Read the model definition and answer for the solid it produces. Units are mm, in the model's axes. A direction names the side the tool comes from. Give positions to 0.01 mm unless a question says otherwise; leave off trailing zeros. Write each loop counter-clockwise with the first axis right and the second up, starting at its lowest first coordinate (ties: lowest second). Pieces come first, ordered by that corner, then holes. Notation, with made-up numbers: (34, 47) -> (50, 47) arc R27 ccw to (50, 68) -> close; hole circle Ø10 at (78.25, 26.25). An arc over 180 degrees is marked (long way). Use a Markdown table: item, result.
from build123d import *

# Parameters (mm, degrees)
SKETCH2_R           = 2.5
BOSS_EXTRUDE1_DEPTH = 3
CUT_EXTRUDE1_START  = -15
CUT_EXTRUDE1_DEPTH  = 15


with BuildPart() as part:
    # Sketch1 → Revolve1 (revolve)
    with BuildSketch(Plane.XY, mode=Mode.PRIVATE) as revolve1_sk:
        Polygon((0, 48.5), (37.1, 48.5), (37.1, 4), (82.1, 4), (82.1, 2.5), (94.1, 2.5), (94.1, 0), (-101.4, 0), (-101.4, 2.4), (-89.4, 2.4), (-89.4, 4), (-38.4, 4), (-38.4, 48.5), align=None)
    revolve(revolve1_sk.sketch.rotate(Axis((0, 0, 0), (-1, 0, 0)), 90), axis=Axis((0, 0, 0), (-1, 0, 0)))

    # Sketch2 → Boss-Extrude1 (add)
    with BuildSketch(Plane(origin=(0, 0, 0), x_dir=(0, 0, -1), z_dir=(1, 0, 0))):
        with BuildLine():
            Line((-7.930604102, 69.771502825), (-16.421800454, 47.75536064))
            ThreePointArc((-16.421800454, 47.75536064), (-43.734282891, 25.25), (-49.568255708, -9.655983951))
            Line((-49.568255708, -9.655983951), (-64.389195958, -28.017646793))
            ThreePointArc((-64.389195958, -28.017646793), (-65.136215932, -37.606411802), (-56.458591856, -41.753856033))
            Line((-56.458591856, -41.753856033), (-33.146455254, -38.099376689))
            ThreePointArc((-33.146455254, -38.099376689), (0, -50.5), (33.146455254, -38.099376689))
            Line((33.146455254, -38.099376689), (56.458591856, -41.753856033))
            ThreePointArc((56.458591856, -41.753856033), (65.136215932, -37.606411802), (64.389195958, -28.017646793))
            Line((64.389195958, -28.017646793), (49.568255708, -9.655983951))
            ThreePointArc((49.568255708, -9.655983951), (43.734282891, 25.25), (16.421800454, 47.75536064))
            Line((16.421800454, 47.75536064), (7.930604102, 69.771502825))
            ThreePointArc((7.930604102, 69.771502825), (0, 75.212823605), (-7.930604102, 69.771502825))
        make_face()
        with Locations((0, 66.712823605)):
            Circle(SKETCH2_R, mode=Mode.SUBTRACT)
        with Locations((57.775, -33.356411802)):
            Circle(SKETCH2_R, mode=Mode.SUBTRACT)
        with Locations((-57.775, -33.356411802)):
            Circle(SKETCH2_R, mode=Mode.SUBTRACT)
    extrude(amount=BOSS_EXTRUDE1_DEPTH)

    # Sketch4 → Cut-Extrude1 (cut)
    with BuildSketch(Plane.ZY.offset(89.4).offset(CUT_EXTRUDE1_START)):
        with BuildLine():
            Line((-2.645751311, 3), (2.645751311, 3))
            ThreePointArc((2.645751311, 3), (0, 4), (-2.645751311, 3))
        make_face()
    extrude(amount=CUT_EXTRUDE1_DEPTH, mode=Mode.SUBTRACT)


solid = part.part
Item 1: Straight lines are drawn through the part: line 1 along X through (y, z) = (19, 17.5); line 2 along X through (y, z) = (-31, 45); line 3 along Z through (x, y) = (33, 38). For each, find the intervals that lie inside material, in ascending order. Write a range as [from, to].
Return value:
| item | result |
|---|---|
| line 1 | [-38.4, 37.1] |
| line 2 | [0, 3] |
| line 3 | [-30.14, 30.14] |
Item 2: A cutting plane is placed at C-C (z = 40). Give the vertices of the cut face in (x, y).
Return value:
| item | result |
|---|---|
| outline | (-38.4, -27.43) -> (0, -27.43) -> (0, -39.17) -> (3, -39.17) -> (3, -27.43) -> (37.1, -27.43) -> (37.1, 27.43) -> (3, 27.43) -> (3, 30.83) -> (0, 30.83) -> (0, 27.43) -> (-38.4, 27.43) -> close |
Item 3: Each of these flat-tipped pins is pushed along its axis until it touches: P1, Ø4.5, axis at y = 66.71, z = 0, coming from the +X side; P2, Ø8, axis at y = -33.36, z = 57.78, coming from the -X side; P3, Ø12, axis at x = 40.5, z = 45.5, coming from the +Y side; P4, Ø4, axis at x = -85, z = -0.5, coming from the +Y side. Where does it stop, or does it pass through?
Return value:
| item | result |
|---|---|
| P1 | through |
| P2 | x = 0 |
| P3 | y = 26.6 |
| P4 | y = 3 |
Item 4: A cutting plane is placed at B-B (y = 0). Give the vertices of the cut face in (x, z).
Return value:
| item | result |
|---|---|
| outline | (-101.4, -2.4) -> (-89.4, -2.4) -> (-89.4, -4) -> (-38.4, -4) -> (-38.4, -48.5) -> (0, -48.5) -> (0, -50.5) -> (3, -50.5) -> (3, -48.5) -> (37.1, -48.5) -> (37.1, -4) -> (82.1, -4) -> (82.1, -2.5) -> (94.1, -2.5) -> (94.1, 2.5) -> (82.1, 2.5) -> (82.1, 4) -> (37.1, 4) -> (37.1, 48.5) -> (3, 48.5) -> (3, 50.5) -> (0, 50.5) -> (0, 48.5) -> (-38.4, 48.5) -> (-38.4, 4) -> (-89.4, 4) -> (-89.4, 2.4) -> (-101.4, 2.4) -> close |
Item 5: A cutting plane is placed at D-D (x = -79). Give the vertices of the cut face in (y, z).
Return value:
| item | result |
|---|---|
| outline | (3, -2.65) -> (3, 2.65) arc R4 ccw (long way) to start |
Item 6: For a pull along Y with two mould halves and no side action, classify faces 1 (the face through (1.48, -31.25, 56.43)), 2 (the face through (-38.4, 10, -1)), 3 (the face through (19.811, 43.028, -22.38)) as +Y half, -Y half, draft (parallel to the pull), parting line (faces both ways), or undercut.
Return value:
| item | result |
|---|---|
| face 1 | undercut |
| face 2 | draft |
| face 3 | parting line |
Item 7: A tool of negligible diameter and unlimited length cuts with its end or side. For faces 4 (the face through (3, 45, 20)), 5 (the face through (-95.316, -2.024, -1.29)), 6 (the face through (-82, 3, 0)), from which of +Z, -Z, +X, -X, +Y, -Y can it reach the whole face along a straight path? Write none if from no direction.
Return value:
| item | result |
|---|---|
| face 4 | +X |
| face 5 | -X |
| face 6 | +Z, -Z, -X, +Y |
